Answer from the drawing. Dimensions are ordinates in mm from the lowest x, y and z of the part. A direction names the side the tool comes from. Round coordinates to 2 decimals unless told otherwise and drop trailing zeros. Write each loop counter-clockwise with the first axis right and the second up, starting at its lowest first coordinate (ties: lowest second). Pieces come first, ordered by that corner, then holes. Notation, with made-up numbers: (73, 43.5) -> (94, 43.5) arc R29 cw to (94, 80.5) -> close; hole circle Ø3 at (10, 23.25). An arc over 180 degrees is marked (long way). Return JSON: item names as keys, results as strings. Group by question number.
(1) For the marked faces 1 and 2, determine the directions among +Z, -Z, +X, -X, +Y, -Y from which every point of the face is accessible in a straight line to the end or side of a thin tool.
(2) A cutting plane is placed at C-C on x = 75. Give the vertices of the cut face in (y, z), then the cut area to 3 significant figures.
(3) A cutting plane is placed at B-B on z = 68. Give the vertices of the cut face in (x, y).
(4) Given pin 1 (6.5 mm diameter, centred on y = 9.5, z = 108, fed in from -X); pin 2 (6 mm diameter, centred on x = 147, z = 137, fed in from +Y), each flat-ended and moving along its own axis, determine where each tip first touches the part or whether it passes through.
(5) A cutting plane is placed at A-A on y = 10. Give the vertices of the cut face in (x, z).
(6) Straight lines are drawn through the part: line 1 (X direction, y = 9, z = 102) (1 decimal); line 2 (Z direction, x = 184, y = 7.75) (1 decimal); line 3 (Z direction, x = 89.5, y = 7.25) (1 decimal). For each, find the intervals that lie inside material, in ascending order.
(7) The mould has two halves that part along Z. Classify the marked faces 3, 4 and 5: released by +Z, released by -Z, zero draft, split by the parting line, or undercut.
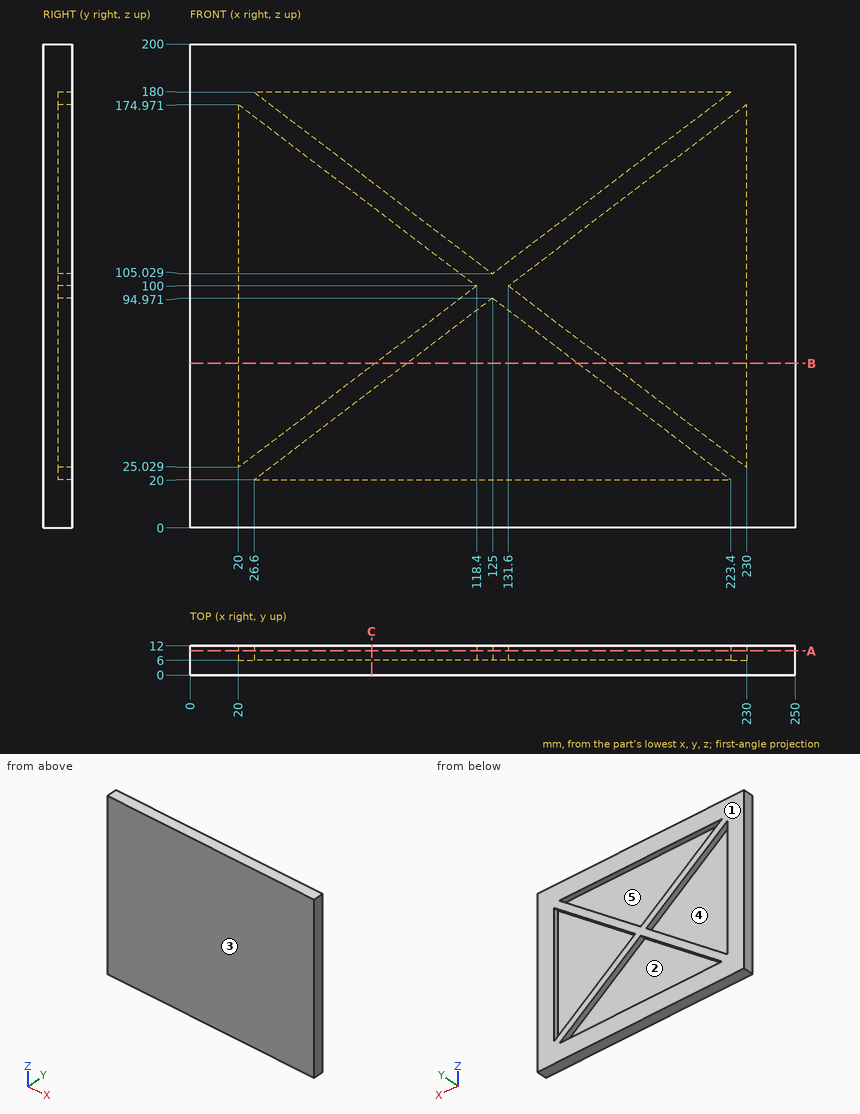
Checks:
{
 "1": {"face 1": "+Z, -Z, +X, -X, +Y", "face 2": "+Y"},
 "2": {"outline": "(0, 0) -> (12, 0) -> (12, 20) -> (6, 20) -> (6, 56.88) -> (12, 56.88) -> (12, 66.93) -> (6, 66.93) -> (6, 133.07) -> (12, 133.07) -> (12, 143.12) -> (6, 143.12) -> (6, 180) -> (12, 180) -> (12, 200) -> (0, 200) -> close", "area": "1,560 mm^2"},
 "3": {"outline": "(0, 0) -> (250, 0) -> (250, 12) -> (230, 12) -> (230, 6) -> (173.6, 6) -> (173.6, 12) -> (160.4, 12) -> (160.4, 6) -> (89.6, 6) -> (89.6, 12) -> (76.4, 12) -> (76.4, 6) -> (20, 6) -> (20, 12) -> (0, 12) -> close"},
 "4": {"pin 1": "stops at x = 0", "pin 2": "stops at y = 6"},
 "5": {"outline": "(0, 0) -> (250, 0) -> (250, 200) -> (0, 200) -> close; hole (20, 25.03) -> (118.4, 100) -> (20, 174.97) -> close; hole (26.6, 20) -> (223.4, 20) -> (125, 94.97) -> close; hole (26.6, 180) -> (125, 105.03) -> (223.4, 180) -> close; hole (131.6, 100) -> (230, 25.03) -> (230, 174.97) -> close"},
 "6": {"line 1": "x = 0 to 20, 115.8 to 134.2, 230 to 250", "line 2": "z = 0 to 20, 50 to 60.1, 139.9 to 150, 180 to 200", "line 3": "z = 0 to 20, 67.9 to 78, 122 to 132.1, 180 to 200"},
 "7": {"face 3": "zero draft", "face 4": "undercut", "face 5": "undercut"}
}
